```python
from build123d import *

# Parameters (mm, degrees)
SKETCH4_R                    = 13.7795
BOSS_EXTRUDE1_DEPTH          = 25.4
SKETCH5_R                    = 13.7795
BOSS_EXTRUDE2_DEPTH          = 12.7
F_3_8_0_375_DIAMETER_HOLE1_D = 9.525


with BuildPart() as part:
    # Sketch1 → Revolve1 (revolve)
    with BuildSketch(Plane.XY):
        Polygon((-31.75, -13.7795), (-12.7, -13.7795), (-12.7, -10.6172), (-31.75, -10.7696), align=None)
        Polygon((31.75, -10.7696), (12.7, -10.6172), (12.7, -13.7795), (31.75, -13.7795), align=None)
    revolve(axis=Axis((-31.75, 0, 0), (1, 0, 0)))



with BuildPart() as body_2:
    # Sketch2 → Revolve2 (revolve)
    with BuildSketch(Plane.XY):
        Polygon((10.7696, 31.75), (10.6172, 12.7), (13.7795, 12.7), (13.7795, 31.75), align=None)
    revolve(axis=Axis((0, 0, 0), (0, 1, 0)))


with BuildPart() as part_1:
    add(part.part)

    add(body_2.part)  # Boss-Extrude1 merges body 2
    # Sketch4 → Boss-Extrude1 (add)
    with BuildSketch(Plane(origin=(-12.7, 0, 0), x_dir=(0, 0, -1), z_dir=(1, 0, 0))):
        Circle(SKETCH4_R)
    extrude(amount=BOSS_EXTRUDE1_DEPTH)

    # Sketch5 → Boss-Extrude2 (add)
    with BuildSketch(Plane.XZ.offset(-12.7)):
        Circle(SKETCH5_R)
    extrude(amount=BOSS_EXTRUDE2_DEPTH)

    # Sketch6 → Cut-Revolve1 (revolve, cut)
    with BuildSketch(Plane.XY):
        Polygon((-31.75, -10.7696), (-12.7, -10.6172), (-12.7, -7.8994), (12.7, -7.8994), (12.7, -10.6172), (31.75, -10.7696), (31.75, 0), (-31.75, 0), align=None)
    revolve(axis=Axis((31.75, 0, 0), (-1, 0, 0)), mode=Mode.SUBTRACT)

    # Sketch7 → Cut-Revolve2 (revolve, cut)
    with BuildSketch(Plane.XY):
        Polygon((10.7696, 31.75), (10.6172, 12.7), (7.8994, 12.7), (7.8994, 0), (0, 0), (0, 31.75), align=None)
    revolve(axis=Axis((0, 0, 0), (0, 1, 0)), mode=Mode.SUBTRACT)

    # 3/8 (0.375) Diameter Hole1 (through all)
    with Locations(Plane(origin=(0, 31.75, 0), x_dir=(-1, 0, 0), z_dir=(0, 1, 0))):
        with Locations((0, 0)):
            Hole(F_3_8_0_375_DIAMETER_HOLE1_D / 2)


solid = part_1.part
```
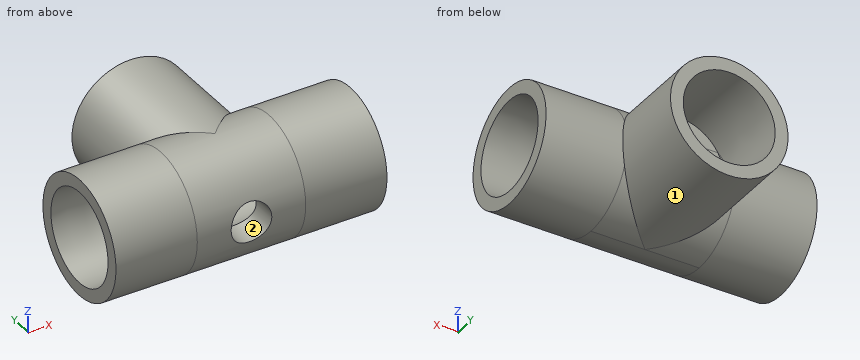
Geometry check sheet. Reference: the model listing, model coordinates, mm. Face numbers are marked on the shaded views. Give positions to 0.01 mm unless a question says otherwise; leave off trailing zeros. Order: outer loops, then holes, each group sorted by start corner. A loop starts at its lowest first (then second) coordinate and runs counter-clockwise, first axis right, second up.
1. Gauge pin test, flat ends, axial feed: pin 1 Ø14 at (x, z) = (0, 0) entering from +Y; pin 2 Ø1.5 at (x, z) = (-16, -9) entering from +Y; pin 3 Ø16 at (y, z) = (-2, 1.5) entering from -X. Record the tip position at first contact, or that the pin passes through.
2. Section check C-C, the plane x = -17. Enter the section's corners in (y, z).
3. Section check A-A, the plane y = 12. Enter the section's corners in (x, z).
4. Section check B-B, the plane z = 2.5. Give the number of separate pieces and of enclosed holes in the cut face, and give its area (3 significant figures).
5. Release check for a two-part mould opening along Z. For the marked faces 1 and 2 record: pulls with the +Z half, pulls with the -Z half, needs draft (parallel to the pull), parting line crosses it, or undercut.
6. Thickness scan on L1, parallel to Z at x = 1.75, y = 0; L2, parallel to X at y = -10.5, z = 0; L3, parallel to X at y = 9.25, z = 0. Record the ranges inside material, lowest first.
Values follow:
1. pin 1: stops at y = -3.66
1. pin 2: stops at y = 11.04
1. pin 3: stops at x = -12.7
2. outline: circle Ø27.56 at (0, 0); hole circle Ø21.3 at (0, 0)
3. outline: (-31.75, -6.77) - (-12, -6.77) arc R13.78 ccw to (12, -6.77) - (31.75, -6.77) - (31.75, 6.77) - (12, 6.77) arc R13.78 ccw to (-12, 6.77) - (-31.75, 6.77) - close; hole circle Ø15.8 at (0, 0)
4. separate pieces: 4
4. enclosed holes: 0
4. area: 518 mm2
5. face 1: parting line crosses it
5. face 2: undercut
6. L1: z = -13.78 to -7.9, 7.9 to 13.78
6. L2: x = -12.7 to -4.76, 4.76 to 12.7
6. L3: x = -12.7 to -7.9, 7.9 to 12.7
